For this review, take the finished solid that the model builds, in its own axes (mm). Face numbers are marked on the shaded views. Coordinates: 2 decimals unless noted, no trailing zeros. Write each loop counter-clockwise with the first axis right and the second up, starting at its lowest first coordinate (ties: lowest second). Pieces come first, ordered by that corner, then holes. Notation, with made-up numbers: (19.25, 9.5) -> (38.25, 9.5) arc R27 ccw to (38.25, 25.5) -> close; hole circle Ø4 at (8.25, 47). An arc over 180 degrees is marked (long way). One line per item, written item: value. Start each with the question number.
1) Add section B-B (x = 0). State the section outline as (y, z) points, and give its area (3 significant figures).
2) For probe 1 along Y at (x, z) = (0, 3.95); probe 2 along X at (y, z) = (-3.25, 3.4), list the stretches that pass through material, from the lowest coordinate up. Write a range as from..to.
3) Add section C-C (x = -3.5). State the section outline as (y, z) points.
4) Add section D-D (z = 4.1). State the section outline as (x, y) points.
5) Mouldability with a two-part tool opening along X and no side actions: class the marked faces 1 and 2 as released by +X, released by -X, zero draft, split by the parting line, or undercut.
6) Add section A-A (y = 0.25). State the section outline as (x, z) points, and give its area (3 significant figures).
7) For pin 1 Ø1.2 at (y, z) = (2, 1) entering from +X; pin 2 Ø0.7 at (y, z) = (4, 1) entering from -X, all flat-tipped, find the tip position at first contact; note any pin that passes through.
from build123d import *

# Parameters (mm, degrees)
SKETCH2_R           = 4.4
SKETCH2_R_2         = 3.75
BOSS_EXTRUDE1_DEPTH = 5
CUT_EXTRUDE1_DEPTH  = 5


with BuildPart() as part:
    # Sketch2 → Boss-Extrude1 (new body)
    with BuildSketch(Plane.XY):
        Circle(SKETCH2_R)
        Circle(SKETCH2_R_2, mode=Mode.SUBTRACT)
    extrude(amount=BOSS_EXTRUDE1_DEPTH)

    # Sketch3 → Cut-Extrude1 (cut)
    with BuildSketch(Plane(origin=(0, 4.4, 0), x_dir=(1, 0, 0), z_dir=(0, 1, 0))):
        Polygon((1.05, -5), (3.25, -5), (3.25, -3.60176001), (-1.05, -1.4), (-1.05, 0), (-3.25, 0), (-3.25, -1.4), (1.05, -3.60176001), align=None)
    extrude(amount=-CUT_EXTRUDE1_DEPTH, mode=Mode.SUBTRACT)


solid = part.part
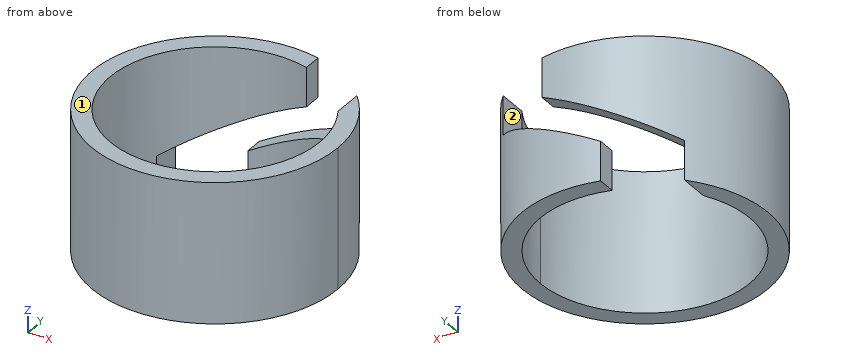
Numbers:
1. outline: (-4.4, 0) -> (-3.75, 0) -> (-3.75, 5) -> (-4.4, 5) -> close; (3.75, 0) -> (4.4, 0) -> (4.4, 1.94) -> (3.75, 1.94) -> close; (3.75, 3.06) -> (4.4, 3.06) -> (4.4, 5) -> (3.75, 5) -> close
1. area: 5.77 mm²
2. probe 1: -4.4..-3.75, 3.75..4.4
2. probe 2: -2.97..-1.87, 1.87..2.97
3. outline: (-2.67, 0) -> (-1.35, 0) -> (-1.35, 5) -> (-2.67, 5) -> close; (1.35, 0) -> (2.67, 0) -> (2.67, 5) -> (1.35, 5) -> close
4. outline: (1.05, 3.6) -> (1.05, 4.27) arc R4.4 ccw (long way) to (3.25, 2.97) -> (3.25, 1.87) arc R3.75 cw (long way) to start
5. face 1: zero draft
5. face 2: undercut
6. outline: (-4.39, 0) -> (-3.74, 0) -> (-3.74, 5) -> (-4.39, 5) -> close; (3.74, 0) -> (4.39, 0) -> (4.39, 5) -> (3.74, 5) -> close
6. area: 6.51 mm²
7. pin 1: x = 4.17
7. pin 2: x = -1.05
